from build123d import *

# Parameters (mm, degrees)
F0_W     = 9.5
F0_H     = 4
F1_DEPTH = 3.5
F2_R     = 1.74999
F3_R     = 0.75
F4_DEPTH = 10
F5_W     = 2.5
F5_H     = 32
F6_DEPTH = 17.5
F7_W     = 14.4
F7_H     = 32
F8_DEPTH = 2.5
F9_R     = 5
F10_SIZE = 1


# Not quite as in the source:
# - a fillet or chamfer is up to 0.001 mm smaller than in the source, because OpenCascade refuses the exact size


with BuildPart() as f1:
    # F0 (on Top) → F1 (new body)
    with BuildSketch(Plane.XY):
        Polygon((0, 40), (0, 0), (35, 0), (35, 40), (22.25, 40), (12.75, 40), align=None)
        with Locations((17.5, 42)):
            Rectangle(F0_W, F0_H)
    extrude(amount=F1_DEPTH)

    # F2 (radius 1.75 in the source; OpenCascade refuses exactly that, so slightly less here)
    f2_edges = [f1.edges().sort_by_distance(p)[0] for p in [
        (17.5, 44, 3.5),
        (17.5, 44, 0),
    ]]
    fillet(f2_edges, radius=F2_R)

    # F3 (on face) → F4 (cut)
    with BuildSketch(Plane.YZ.offset(22.25)):
        with Locations((42.25, 1.75)):
            Circle(F3_R)
    extrude(amount=-F4_DEPTH, mode=Mode.SUBTRACT)

    # F5 (on face) → F6 (join)
    with BuildSketch(Plane.XY.offset(3.5)):
        with Locations((11.55, 16)):
            Rectangle(F5_W, F5_H)
        with Locations((23.45, 16)):
            Rectangle(F5_W, F5_H)
    extrude(amount=F6_DEPTH)

    # F7 (on face) → F8 (join)
    with BuildSketch(Plane.XY.offset(21)):
        with Locations((17.5, 16)):
            Rectangle(F7_W, F7_H)
    extrude(amount=F8_DEPTH)

    # F9
    f9_edges = [f1.edges().sort_by_distance(p)[0] for p in [
        (24.7, 16, 23.5),
        (10.3, 16, 23.5),
        (24.7, 16, 3.5),
        (10.3, 16, 3.5),
        (35, 40, 1.75),
        (0, 40, 1.75),
        (0, 0, 1.75),
        (35, 0, 1.75),
    ]]
    fillet(f9_edges, radius=F9_R)

    # F10
    f10_edges = [f1.edges().sort_by_distance(p)[0] for p in [
        (12.8, 0, 12.25),
        (17.5, 0, 3.5),
        (22.2, 0, 12.25),
        (17.5, 0, 21),
    ]]
    chamfer(f10_edges, length=F10_SIZE)


solid = f1.part
Geometry: final body of the model. Coordinates: model frame, mm. A direction names the side the tool comes from. Give positions to 0.01 mm unless a question says otherwise; leave off trailing zeros. Write each loop counter-clockwise with the first axis right and the second up, starting at its lowest first coordinate (ties: lowest second). Pieces come first, ordered by that corner, then holes. Notation, with made-up numbers: (84.25, -13) - (115.25, -13) arc R18 cw to (115.25, 19) - close; hole circle Ø11 at (21, -34.75). An arc over 180 degrees is marked (long way). Return JSON: item names as keys, results as strings. Group by question number.
1) Section B-B on x = 13.5. State how many separate pieces and enclosed holes the cut face has, plus the area to 3 significant figures.
2) Set-up query: faces 5 (the flat face through (17, 17, 21)), 6 (the flat face through (22.25, 41, 2)), 7 (the flat face through (17.4, 0.5, 21.5)), 8 (the flat face through (10.3, 16, 13)). Return all of +Z, -Z, +X, -X, +Y, -Y with unobstructed straight access to the full face (end or side cutting, diameter ignored); none if empty.
3) Section C-C on z = 12. Return the cut outline in (x, y), plus the area to 3 significant figures.
4) Section D-D on x = 26.5. Return the cut outline in (y, z), plus the area to 3 significant figures.
5) Line query: line 1 (Z direction, x = 16, y = 42.25); line 2 (X direction, y = 7, z = 11.5); line 3 (Z direction, x = 16, y = 31.5). Output: solid intervals per line, ascending.
6) Section A-A on y = 5.5. Return the cut outline in (x, z).
7) First-contact query: P1, Ø5, axis at y = 15, z = 14, coming from the +X side; P2, Ø3, axis at y = 42, z = 1.5, coming from the -X side; P3, Ø4, axis at y = 32.5, z = 10.5, coming from the -X side. Flat tips, straight axial feed; report the tip coordinate or a pass-through.
8) Mould query, pull axis X, two halves, no side actions, for faces 1 (the flat face through (17, 21, 3.5)), 2 (the flat face through (24.7, 16, 13)), 3 (the flat face through (9, 40, 2)), 4 (the cylindrical face through (2, 1, 2)). Classes: released by +X, released by -X, zero draft, split by the parting line, or undercut.
Filled in:
{
 "1": {"separate pieces": "2", "enclosed holes": "1", "area": "219 mm^2"},
 "2": {"face 5": "+Y, -Y", "face 6": "+Z, -Z, +X, +Y", "face 7": "-Y", "face 8": "+Z, -X, +Y, -Y"},
 "3": {"outline": "(10.3, 0) - (11.8, 0) - (12.8, 1) - (12.8, 32) - (10.3, 32) - close; (22.2, 1) - (23.2, 0) - (24.7, 0) - (24.7, 32) - (22.2, 32) - close", "area": "159 mm^2"},
 "4": {"outline": "(0, 0) - (40, 0) - (40, 3.5) - (32, 3.5) - (32, 4.66) - (0, 4.66) - close", "area": "177 mm^2"},
 "5": {"line 1": "z = 0 to 1, 2.5 to 3.5", "line 2": "x = 10.3 to 12.8, 22.2 to 24.7", "line 3": "z = 0 to 3.5, 21 to 23.5"},
 "6": {"outline": "(0, 0) - (35, 0) - (35, 3.5) - (29.7, 3.5) arc R5 cw to (24.7, 8.5) - (24.7, 18.5) arc R5 ccw to (19.7, 23.5) - (15.3, 23.5) arc R5 ccw to (10.3, 18.5) - (10.3, 8.5) arc R5 cw to (5.3, 3.5) - (0, 3.5) - close; hole (12.8, 3.5) - (22.2, 3.5) - (22.2, 21) - (12.8, 21) - close"},
 "7": {"P1": "stops at x = 24.7", "P2": "stops at x = 12.75", "P3": "stops at x = 10.3"},
 "8": {"face 1": "undercut", "face 2": "released by +X", "face 3": "zero draft", "face 4": "released by -X"}
}
